from build123d import *

# Parameters (mm, degrees)
F0_W     = 50.8
F0_H     = 50.8
F0_W_2   = 47.625
F0_H_2   = 47.625
F1_DEPTH = 895.35
F2_R     = 3.175
F3_R     = 1.5875


with BuildPart() as f1:
    # F0 (on Top) → F1 (new body)
    with BuildSketch(Plane.XY):
        with Locations((-12.7, -11.264074)):
            Rectangle(F0_W, F0_H)
        with Locations((-12.7, -11.264074)):
            Rectangle(F0_W_2, F0_H_2, mode=Mode.SUBTRACT)
    extrude(amount=-F1_DEPTH)

    # F2
    f2_edges = [f1.edges().sort_by_distance(p)[0] for p in [
        (-38.1, -36.664074, -447.675),
        (12.7, -36.664074, -447.675),
        (12.7, 14.135926, -447.675),
        (-38.1, 14.135926, -447.675),
    ]]
    fillet(f2_edges, radius=F2_R)

    # F3
    f3_edges = [f1.edges().sort_by_distance(p)[0] for p in [
        (-36.5125, 12.548426, -447.675),
        (11.1125, 12.548426, -447.675),
        (11.1125, -35.076574, -447.675),
        (-36.5125, -35.076574, -447.675),
    ]]
    fillet(f3_edges, radius=F3_R)


solid = f1.part
Here's how the part is built. I have some questions about the finished solid (model axes, mm). A direction names the side the tool comes from. Coordinates: 2 decimals unless noted, no trailing zeros. Order: outer loops, then holes, each group sorted by start corner. A loop starts at its lowest first (then second) coordinate and runs counter-clockwise, first axis right, second up.
Item 1: If we section it at A-A on y = -12: List the corners of the cut face in (x, z) for me, plus the area to 3 significant figures.
Result sheet:
outline: (-38.1, -895.35) - (-36.51, -895.35) - (-36.51, 0) - (-38.1, 0) - close; (11.11, -895.35) - (12.7, -895.35) - (12.7, 0) - (11.11, 0) - close
area: 2,840 mm2
Item 2: For P1, Ø4, axis at x = 1, y = 9, coming from the +Z side, with a flat end and sliding along its axis, tell me the tip position at first contact or that it passes through.
Result sheet:
P1: passes through
Item 3: If we section it at B-B on x = -18.5: List the corners of the cut face in (y, z) for me.
Result sheet:
outline: (-36.66, -895.35) - (-35.08, -895.35) - (-35.08, 0) - (-36.66, 0) - close; (12.55, -895.35) - (14.14, -895.35) - (14.14, 0) - (12.55, 0) - close
Item 4: For faces 5 (the face through (-36.512, -12, -441)), 6 (the face through (-38.1, -12, -441)), which set-ups out of +Z, -Z, +X, -X, +Y, -Y let a thin tool reach every point of the face, with its end or its side?
Result sheet:
face 5: +Z, -Z
face 6: +Z, -Z, -X, +Y, -Y
Item 5: I need wall thicknesses on line 1 (Y direction, x = -9, z = -572); line 2 (X direction, y = -18, z = -42); line 3 (Y direction, x = -36, z = -613.5). Which ranges of each line are inside material? Lowest first, please.
Result sheet:
line 1: y = -36.66 to -35.08, 12.55 to 14.14
line 2: x = -38.1 to -36.51, 11.11 to 12.7
line 3: y = -36.48 to -34.66, 12.13 to 13.95
Item 6: If we mould it in two halves opening along Y, with no side actions, what happens to faces 1 (the face through (12.7, -12, -441)), 2 (the face through (-13, 14.136, -441)), 3 (the face through (-13, -36.664, -441)), 4 (the face through (-13, -35.077, -441))? For each: +Y half, -Y half, draft (parallel to the pull), parting line (faces both ways), or undercut.
Result sheet:
face 1: draft
face 2: +Y half
face 3: -Y half
face 4: undercut
